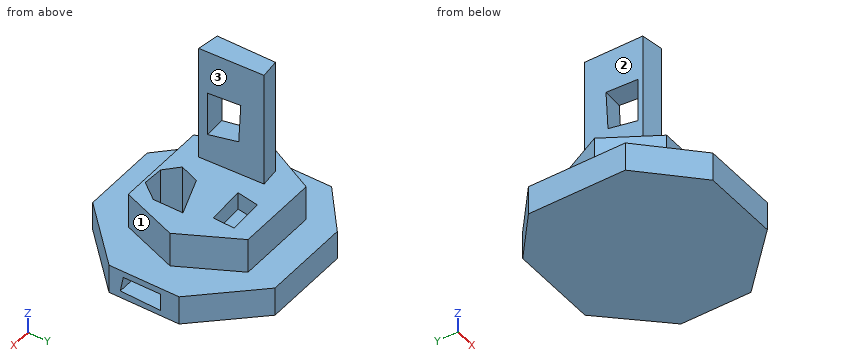
from build123d import *

# Parameters (mm, degrees)
PAD_DEPTH       = 10
PAD001_DEPTH    = 12
PAD002_DEPTH    = 40
POCKET_DEPTH    = 6
POCKET001_DEPTH = 18
POCKET002_DEPTH = 9
POCKET003_DEPTH = 40


with BuildPart() as part:
    # Sketch → Pad (new body)
    with BuildSketch(Plane.XY):
        Polygon((-10.633484, 29.864252), (19.9095, 29.864252), (38.687782, 9.95475), (38.687782, -14.253396), (18.778282, -33.936649), (-7.918551, -33.936649), (-25.791855, -16.289593), (-25.791855, 17.194569), align=None)
    extrude(amount=PAD_DEPTH)

    # Sketch002 (on Face10 of Pad) → Pad001 (join)
    with BuildSketch(Plane.XY.offset(10)):
        Polygon((-9.896216, 19.621426), (18.610573, 19.621426), (29.017811, 0), (21.777992, -19.518847), (-10.12246, -19.518847), (-20.755943, -2.09803), align=None)
    extrude(amount=PAD001_DEPTH)

    # Sketch003 (on Face17 of Pad001) → Pad002 (join)
    with BuildSketch(Plane.XY.offset(22)):
        Polygon((-10.574949, 8.535451), (-4.013864, 9.214187), (-3.108886, -12.731516), (-10.574949, -11.600292), align=None)
    extrude(amount=PAD002_DEPTH)

    # Sketch004 (on Face17 of Pad002) → Pocket (cut)
    with BuildSketch(Plane.XY.offset(22)):
        Polygon((4.578534, 12.919245), (16.729834, 13.542388), (16.418259, 6.064667), (3.332247, 5.441524), align=None)
    extrude(amount=-POCKET_DEPTH, mode=Mode.SUBTRACT)

    # Sketch005 (on Face17 of Pocket) → Pocket001 (cut)
    with BuildSketch(Plane.XY.offset(22)):
        Polygon((5.699865, -7.326652), (19.550392, -2.196826), (19.550392, -12.456478), (14.762555, -18.612268), (7.751796, -18.270281), (3.13495, -13.995423), align=None)
    extrude(amount=-POCKET001_DEPTH, mode=Mode.SUBTRACT)

    # Sketch006 (on Face27 of Pocket001) → Pocket002 (cut)
    with BuildSketch(Plane(origin=(-3.6277283341, -0.1495971367, 0), x_dir=(-0.0412021215, 0.999150832, 0), z_dir=(0.999150832, 0.0412021215, 0))):
        Polygon((-9.565722, 46.86203), (1.548902, 47.375011), (0.864925, 33.695477), (-9.565722, 31.643547), align=None)
    extrude(amount=-POCKET002_DEPTH, mode=Mode.SUBTRACT)

    # Sketch008 (on Face7 of Pocket002) → Pocket003 (cut)
    with BuildSketch(Plane.YZ.offset(38.687782)):
        Polygon((-9.326732, 7.876174), (3.497833, 7.876174), (3.497833, 1.89138), (-10.352697, 2.404365), align=None)
    extrude(amount=-POCKET003_DEPTH, mode=Mode.SUBTRACT)


solid = part.part
Source: CAD feature listing. Evaluate the final solid. Frame: model axes, mm. Face numbers are marked on the shaded views. A direction names the side the tool comes from. Give positions to 0.01 mm unless a question says otherwise; leave off trailing zeros. Write each loop counter-clockwise with the first axis right and the second up, starting at its lowest first coordinate (ties: lowest second). Pieces come first, ordered by that corner, then holes. Notation, with made-up numbers: (-39, 4) -> (-5, 4) arc R14 cw to (-5, 12) -> close; hole circle Ø1 at (64.25, 22.25). An arc over 180 degrees is marked (long way). Write item = value, one per line.
Q1. Reachability of the marked faces 1, 2 and 3 from +Z, -Z, +X, -X, +Y, -Y: full face, straight path, thin tool, end or side. Return the list, or none.
Here are the results:
face_1 = +Z, +X, -Y
face_2 = +Z, -X, +Y, -Y
face_3 = +Z, +X, +Y
Q2. Cut plane B-B on x = 26.5. Return loops of the section in (y, z).
Here are the results:
outline = (-26.3, 0) -> (22.88, 0) -> (22.88, 10) -> (4.75, 10) -> (4.75, 22) -> (-6.79, 22) -> (-6.79, 10) -> (-26.3, 10) -> close; hole (-10.35, 2.4) -> (3.5, 1.89) -> (3.5, 7.88) -> (-9.33, 7.88) -> close
Q3. First-contact query: pin 1 (10 mm diameter, centred on y = -21, z = 18, fed in from -X); pin 2 (10 mm diameter, centred on y = -0.5, z = 42.5, fed in from -X); pin 3 (12 mm diameter, centred on y = 14.5, z = 55, fed in from +X). Flat tips, straight axial feed; report the tip coordinate or a pass-through.
Here are the results:
pin_1 = -12.27
pin_2 = -10.57
pin_3 = -3.98
Q4. Cut plane A-A on z = 12. Return loops of the section in (x, y).
Here are the results:
outline = (-20.76, -2.1) -> (-10.12, -19.52) -> (21.78, -19.52) -> (29.02, 0) -> (18.61, 19.62) -> (-9.9, 19.62) -> close; hole (3.13, -14) -> (7.75, -18.27) -> (14.76, -18.61) -> (19.55, -12.46) -> (19.55, -2.2) -> (5.7, -7.33) -> close
Q5. Cut plane C-C on z = 35.5. Return loops of the section in (x, y), then the cut area to 3 significant figures.
Here are the results:
outline = (-10.57, -11.6) -> (-3.11, -12.73) -> (-3.23, -9.71) -> (-10.57, -10.01) -> close; (-10.57, 0.52) -> (-3.67, 0.8) -> (-4.01, 9.21) -> (-10.57, 8.54) -> close
area = 72.4 mm²
Q6. Line query: line 1 (Z direction, x = 31, y = -21); line 2 (Z direction, x = -11, y = 4); line 3 (Z direction, x = 35.5, y = -2) (3 decimals). Output: solid intervals per line, ascending. Write a range as from..to.
Here are the results:
line_1 = 0..10
line_2 = 0..22
line_3 = 0..2.095, 7.876..10
Q7. Cut plane D-D on x = -19.5. Return loops of the section in (y, z), then the cut area to 3 significant figures.
Here are the results:
outline = (-22.5, 0) -> (22.45, 0) -> (22.45, 10) -> (0.41, 10) -> (0.41, 22) -> (-4.16, 22) -> (-4.16, 10) -> (-22.5, 10) -> close
area = 504 mm²
